Here's how the part is built. I have some questions about the finished solid (model axes, mm). Round coordinates to 2 decimals unless told otherwise and drop trailing zeros. Order: outer loops, then holes, each group sorted by start corner. A loop starts at its lowest first (then second) coordinate and runs counter-clockwise, first axis right, second up. Notation, with made-up numbers: M 64,68.5 L 110,68.5 A26 ccw 110,101.5 Z; hole C 2.25,-38 d8. An arc over 180 degrees is marked long. Write each question's results on one line, items separated by ' | '. Start each with the question number.
Autodesk Inventor part; units mm, degrees
ref_plane "YZ Plane" through (0, 0, 0) normal (1, 0, 0) x (0, 1, 0)
ref_plane "XZ Plane" through (0, 0, 0) normal (0, 1, 0) x (-1, 0, 0)
ref_plane "XY Plane" through (0, 0, 0) normal (0, 0, 1) x (1, 0, 0)
sketch "Sketch1" plane through (0, 0, 0) normal (0, 0, 1) x (1, 0, 0)
  line L0 (0, 0) -> (491.0582, 0)
  line L1 (491.0582, 0) -> (491.0582, 508)
  line L2 (491.0582, 508) -> (0, 508)
  line L3 (0, 508) -> (0, 0)
  dimension "d0" = 491.0582
  dimension "d1" = 508
extrude "Extrusion1" add sketch "Sketch1" along normal blind 6.35
sketch "Sketch2" plane through (0, 0, 6.35) normal (0, 0, 1) x (1, 0, 0)
  line L0 (42.3291, 457.2) -> (448.7291, 457.2)
  line L1 (448.7291, 457.2) -> (448.7291, 50.8)
  line L2 (448.7291, 50.8) -> (42.3291, 50.8)
  line L3 (42.3291, 50.8) -> (42.3291, 457.2)
  line L4 (245.5291, 50.8) -> (245.5291, 0)
  line L5 (0, 0) -> (491.0582, 0)
  line L6 (245.5291, 457.2) -> (245.5291, 508)
  line L7 (491.0582, 508) -> (0, 508)
  line L8 (42.3291, 254) -> (0, 254)
  line L9 (0, 508) -> (0, 0)
  line L10 (448.7291, 254) -> (491.0582, 254)
  line L11 (491.0582, 0) -> (491.0582, 508)
  dimension "d4" = 406.4
  dimension "d5" = 406.4
extrude "Extrusion2" cut sketch "Sketch2" against normal blind 6.35 contours L0 L1 L2 L3
properties part number "window inner"
(1) I want a section at B-B on y = 331.5. Write out the boundary of the cut face in (x, z).
(2) I want a section at A-A on x = 203.5. Write out the boundary of the cut face in (y, z), and give its area (3 significant figures).
(3) Please list where these lines run through material, in increasing order: line 1 (X direction, y = 97, z = 0.75); line 2 (Y direction, x = 263, z = 2.5).
(4) I want a section at C-C on z = 1. Write out the boundary of the cut face in (x, y), and give its area (3 significant figures).
Solutions:
1) outline: M 0,0 L 42.33,0 L 42.33,6.35 L 0,6.35 Z; M 448.73,0 L 491.06,0 L 491.06,6.35 L 448.73,6.35 Z
2) outline: M 0,0 L 50.8,0 L 50.8,6.35 L 0,6.35 Z; M 457.2,0 L 508,0 L 508,6.35 L 457.2,6.35 Z | area: 645 mm^2
3) line 1: 0 to 42.33, 448.73 to 491.06 | line 2: 0 to 50.8, 457.2 to 508
4) outline: M 0,0 L 491.06,0 L 491.06,508 L 0,508 Z; hole M 42.33,50.8 L 448.73,50.8 L 448.73,457.2 L 42.33,457.2 Z | area: 84,300 mm^2
